Geometry: final body of the model. Coordinates: model frame, mm. Coordinates: 2 decimals unless noted, no trailing zeros. Loops run counter-clockwise (first coordinate to the right, second up) from the corner with the lowest first, then second, coordinate; pieces in that order, holes last. Notation, with made-up numbers: (56.5, 28.5) - (77.5, 28.5) arc R15 ccw to (77.5, 49.5) - close; hole circle Ø5 at (73, -17). An arc over 180 degrees is marked (long way). Answer in a Markdown table with one row per item.
Autodesk Inventor part; units mm, degrees
ref_plane "YZ Plane" through (0, 0, 0) normal (1, 0, 0) x (0, 1, 0)
ref_plane "XZ Plane" through (0, 0, 0) normal (0, 1, 0) x (-1, 0, 0)
ref_plane "XY Plane" through (0, 0, 0) normal (0, 0, 1) x (1, 0, 0)
sketch "Sketch1" plane through (0, 0, 0) normal (0, 1, 0) x (-1, 0, 0)
  line L0 (66.675, 57.15) -> (-66.675, 57.15)
  line L1 (-66.675, 57.15) -> (-66.675, -57.15)
  line L2 (-66.675, -57.15) -> (66.675, -57.15)
  line L3 (66.675, -57.15) -> (66.675, 57.15)
  line L4 (66.675, 57.15) -> (-66.675, -57.15) construction
  line L5 (-66.675, 57.15) -> (66.675, -57.15) construction
  line L6 (19.05, 107.95) -> (-19.05, 107.95)
  line L7 (-19.05, 107.95) -> (-19.05, 6.35)
  line L8 (-19.05, 6.35) -> (19.05, 6.35)
  line L9 (19.05, 6.35) -> (19.05, 107.95)
  line L10 (19.05, 107.95) -> (-19.05, 6.35) construction
  line L11 (-19.05, 107.95) -> (19.05, 6.35) construction
  line L12 (0, 57.15) -> (0, -57.15) construction
  line L13 (-98.425, 34.925) -> (98.425, 34.925)
  line L14 (98.425, 34.925) -> (98.425, -12.7)
  line L15 (98.425, -12.7) -> (-98.425, -12.7)
  line L16 (-98.425, -12.7) -> (-98.425, 34.925)
  line L17 (-98.425, 34.925) -> (98.425, -12.7) construction
  line L18 (98.425, 34.925) -> (-98.425, -12.7) construction
  point P0 (0, 0)
  point P1 (19.05, 57.15)
  point P2 (-19.05, 57.15)
  point P3 (0, 11.1125)
  point P4 (66.675, 34.925)
  point P5 (66.675, -12.7)
  point P6 (-66.675, -12.7)
  point P7 (-66.675, 34.925)
  dimension "d0" = 133.35
  dimension "d1" = 114.3
  dimension "d2" = 38.1
  dimension "d3" = 101.6
  dimension "d6" = 196.85
  dimension "d7" = 22.225
  dimension "d8" = 44.45
extrude "Extrusion1" add sketch "Sketch1" along normal blind 3.175 contours L3 L13 L9 L0 | L13 L14 L15 L3 | L3 L15 L1 L13 L7 L8 L9 | L7 L13 L1 L0 | L3 L2 L1 L15 | L15 L16 L13 L1
fillet "Fillet1" radius 3.175 6 edges at (66.675, 1.5875, 34.925) (66.675, 1.5875, -12.7) (-19.05, 1.5875, 6.35) (19.05, 1.5875, 6.35) (-66.675, 1.5875, 34.925) (-66.675, 1.5875, -12.7)
properties part number "Bottom Plate" material "UHMW, White"
(1) Cut plane C-C on x = 73. Output: boundary loops of the cut face in (y, z) (3 decimals).
Verdict:
| item | result |
|---|---|
| outline | (0, -12.7) - (3.175, -12.7) - (3.175, 34.925) - (0, 34.925) - close |
(2) First-contact query: pin 1 Ø1.5 at (x, y) = (76, 1) entering from -Z; pin 2 Ø1.6 at (y, z) = (1, -46.5) entering from +X (3 decimals); pin 3 Ø1.6 at (y, z) = (1.5, 45) entering from -X (3 decimals). Flat tips, straight axial feed; report the tip coordinate or a pass-through.
Verdict:
| item | result |
|---|---|
| pin 1 | stops at z = -12.7 |
| pin 2 | stops at x = 66.675 |
| pin 3 | stops at x = -66.675 |
(3) Cut plane D-D on z = -47. Output: boundary loops of the cut face in (x, y) (3 decimals), then the cut area to 3 significant figures.
Verdict:
| item | result |
|---|---|
| outline | (-66.675, 0) - (66.675, 0) - (66.675, 3.175) - (-66.675, 3.175) - close |
| area | 423 mm² |
(4) Cut plane A-A on z = 41.5. Output: boundary loops of the cut face in (x, y) (3 decimals), then the cut area to 3 significant figures.
Verdict:
| item | result |
|---|---|
| outline | (-66.675, 0) - (-19.05, 0) - (-19.05, 3.175) - (-66.675, 3.175) - close; (19.05, 0) - (66.675, 0) - (66.675, 3.175) - (19.05, 3.175) - close |
| area | 302 mm² |
(5) Cut plane B-B on y = 2.45. Output: boundary loops of the cut face in (x, z) (3 decimals).
Verdict:
| item | result |
|---|---|
| outline | (-98.425, -12.7) - (-69.85, -12.7) arc R3.175 cw to (-66.675, -15.875) - (-66.675, -57.15) - (66.675, -57.15) - (66.675, -15.875) arc R3.175 cw to (69.85, -12.7) - (98.425, -12.7) - (98.425, 34.925) - (69.85, 34.925) arc R3.175 cw to (66.675, 38.1) - (66.675, 57.15) - (19.05, 57.15) - (19.05, 9.525) arc R3.175 cw to (15.875, 6.35) - (-15.875, 6.35) arc R3.175 cw to (-19.05, 9.525) - (-19.05, 57.15) - (-66.675, 57.15) - (-66.675, 38.1) arc R3.175 cw to (-69.85, 34.925) - (-98.425, 34.925) - close |
(6) Ray query, probe 1 along X at (y, z) = (1.75, 19.5) (3 decimals); probe 2 along Z at (x, y) = (2.5, 1.35); probe 3 along Z at (x, y) = (-75, 1.85) (3 decimals). Return the intervals inside material, ascending.
Verdict:
| item | result |
|---|---|
| probe 1 | x = -98.425 to -19.05, 19.05 to 98.425 |
| probe 2 | z = -57.15 to 6.35 |
| probe 3 | z = -12.7 to 34.925 |
